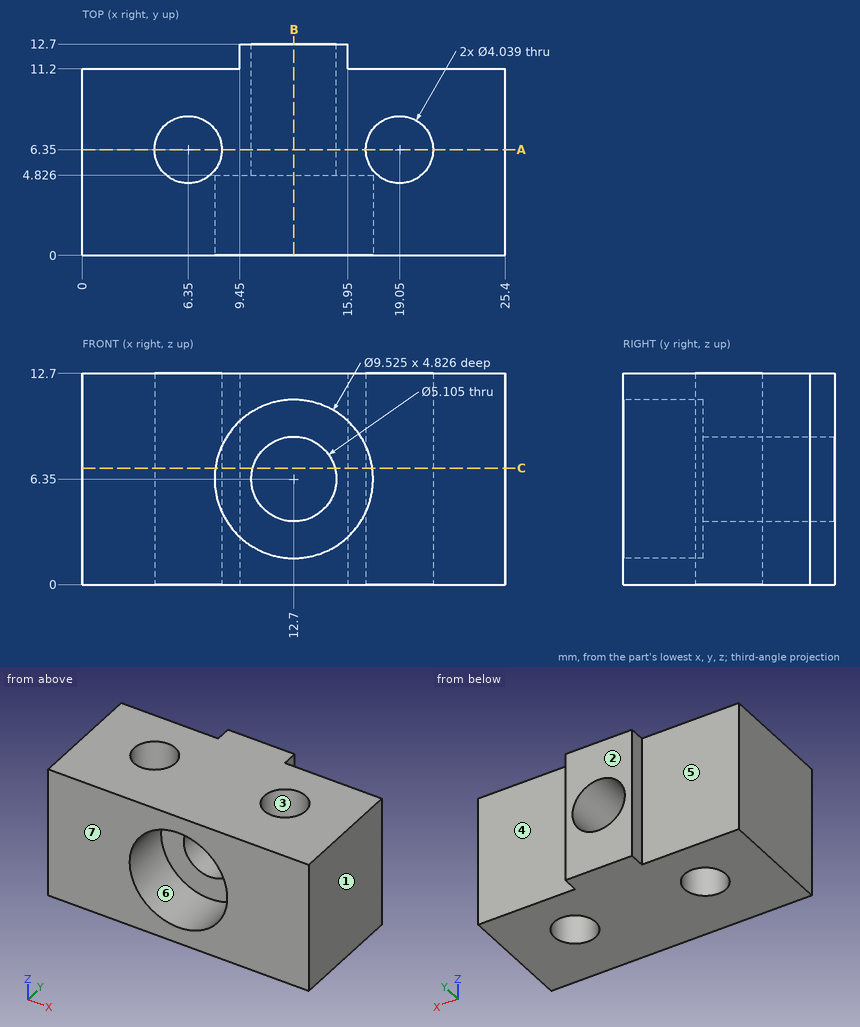
Check sheet for the drawn part. Datum: minimum x, y, z corner. Units: mm. A direction names the side the tool comes from. Round coordinates to 2 decimals unless told otherwise and drop trailing zeros. Order: outer loops, then holes, each group sorted by start corner. A loop starts at its lowest first (then second) coordinate and runs counter-clockwise, first axis right, second up.
(1) Access from +Z, -Z, +X, -X, +Y, -Y to the whole of each face (thin tool, end or side, straight path). Record for the marked faces 4, 5, 6 and 7.
(2) Draft check along X on the marked faces 1, 2 and 3. Enter one of: pulls with the +X half, pulls with the -X half, needs draft (parallel to the pull), parting line crosses it, or undercut.
(3) Cross-section at B-B, the plane x = 12.7. Enter the section's corners in (y, z).
(4) Cross-section at C-C, the plane z = 7. Enter the section's corners in (x, y).
(5) Scan lines: probe 1 along X at (y, z) = (5.5, 11); probe 2 along X at (y, z) = (7.5, 2.75); probe 3 along Z at (x, y) = (12.7, 1.6). Record each from-to range of solid material in increasing order.
(6) Cross-section at A-A, the plane y = 6.35. State how many separate pieces and enclosed holes the cut face has.
(7) Go/stop test with flat-tipped pins: P1, Ø3, axis at x = 19, z = 10.5, coming from the +Y side; P2, Ø5, axis at x = 12.5, z = 6.5, coming from the -Y side; P3, Ø1.2, axis at y = 12, z = 4.5, coming from the -X side. Record where each tip stops, or that it passes through.
Check sheet entries:
1. face 4: +Z, -Z, +X, +Y
1. face 5: +Z, -Z, -X, +Y
1. face 6: -Y
1. face 7: +Z, -Z, +X, -X, -Y
2. face 1: pulls with the +X half
2. face 2: needs draft
2. face 3: undercut
3. outline: (0, 0) - (12.7, 0) - (12.7, 3.8) - (4.83, 3.8) - (4.83, 1.59) - (0, 1.59) - close; (0, 11.11) - (4.83, 11.11) - (4.83, 8.9) - (12.7, 8.9) - (12.7, 12.7) - (0, 12.7) - close
4. outline: (0, 0) - (7.98, 0) - (7.98, 4.83) - (10.23, 4.83) - (10.23, 12.7) - (9.45, 12.7) - (9.45, 11.2) - (0, 11.2) - close; (15.17, 4.83) - (17.42, 4.83) - (17.42, 0) - (25.4, 0) - (25.4, 11.2) - (15.95, 11.2) - (15.95, 12.7) - (15.17, 12.7) - close; hole circle Ø4.04 at (6.35, 6.35); hole circle Ø4.04 at (19.05, 6.35)
5. probe 1: x = 0 to 4.52, 8.18 to 17.22, 20.88 to 25.4
5. probe 2: x = 0 to 4.69, 8.01 to 17.39, 20.71 to 25.4
5. probe 3: z = 0 to 1.59, 11.11 to 12.7
6. separate pieces: 3
6. enclosed holes: 1
7. P1: stops at y = 11.2
7. P2: stops at y = 4.83
7. P3: stops at x = 9.45
